Answer from the drawing. Dimensions are ordinates in mm from the lowest x, y and z of the part. Coordinates: 2 decimals unless noted, no trailing zeros. Order: outer loops, then holes, each group sorted by start corner. A loop starts at its lowest first (then second) coordinate and runs counter-clockwise, first axis right, second up. Notation, with made-up numbers: M 79.25,0 L 101.25,0 A20 cw 101.25,23 Z; hole C 69.25,79 d2. An arc over 180 degrees is marked long. Write each question's results on one line, items separated by ' | '.
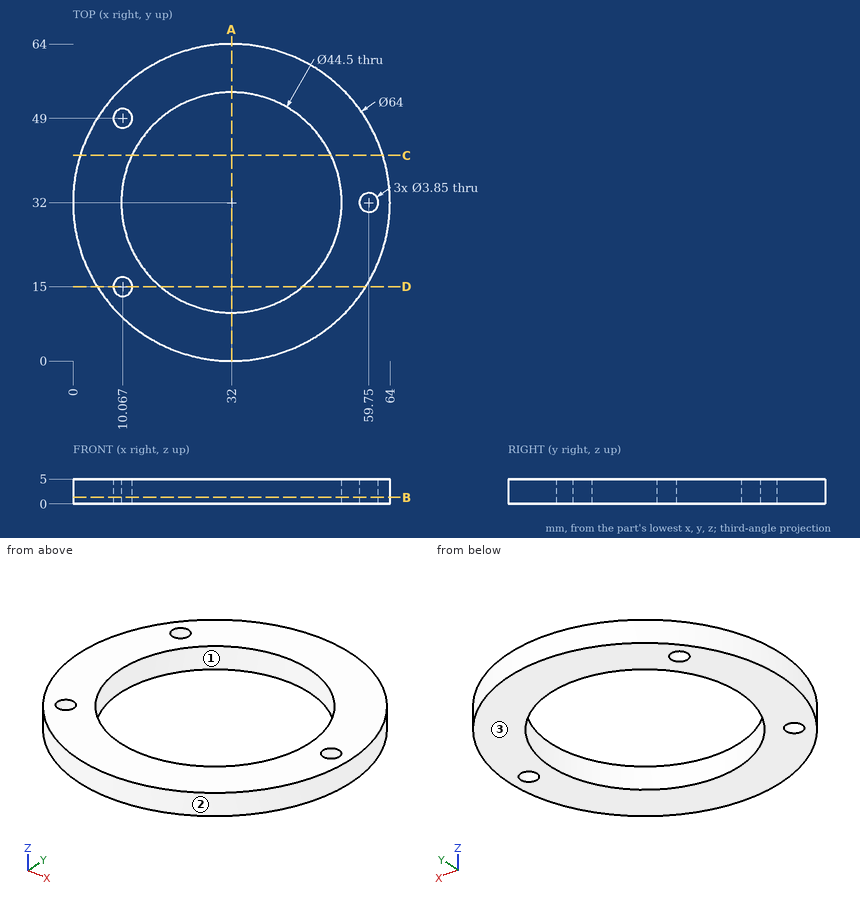
(1) Given pin 1 (2 mm diameter, centred on y = 23.5, z = 2.5, fed in from -X); pin 2 (3 mm diameter, centred on x = 39.5, z = 1, fed in from +Y); pin 3 (1 mm diameter, centred on y = 16, z = 3, fed in from +X), each flat-ended and moving along its own axis, determine where each tip first touches the part or whether it passes through.
Conclusion:
pin 1: x = 0.89 | pin 2: y = 63.43 | pin 3: x = 60
(2) The part is cut by section C-C, the plane y = 41.5. Write down the section's boundary in (x, z).
Conclusion:
outline: M 1.44,0 L 11.88,0 L 11.88,5 L 1.44,5 Z; M 52.12,0 L 62.56,0 L 62.56,5 L 52.12,5 Z
(3) The part is cut by section D-D, the plane y = 15. Write down the section's boundary in (x, z) (3 decimals).
Conclusion:
outline: M 4.889,0 L 8.142,0 L 8.142,5 L 4.889,5 Z; M 11.992,0 L 17.645,0 L 17.645,5 L 11.992,5 Z; M 46.355,0 L 59.111,0 L 59.111,5 L 46.355,5 Z
(4) Straight lines are drawn through the part: line 1 (X direction, y = 49.5, z = 3.5) (1 decimal); line 2 (Y direction, x = 45.5, z = 3.75); line 3 (Y direction, x = 43, z = 0.75). For each, find the intervals that lie inside material, in ascending order.
Conclusion:
line 1: 5.2 to 8.2, 11.9 to 18.3, 45.7 to 58.8 | line 2: 2.99 to 14.31, 49.69 to 61.01 | line 3: 1.95 to 12.66, 51.34 to 62.05
(5) The part is cut by section B-B, the plane z = 1.3. Write down the section's boundary in (x, y) (3 decimals), then the cut area to 3 significant figures.
Conclusion:
outline: C 32,32 d64; hole C 10.067,15 d3.85; hole C 10.067,49 d3.85; hole C 32,32 d44.5; hole C 59.75,32 d3.85 | area: 1,630 mm²
(6) The part is cut by section A-A, the plane x = 32. Write down the section's boundary in (y, z), then the cut area to 3 significant figures.
Conclusion:
outline: M 0,0 L 9.75,0 L 9.75,5 L 0,5 Z; M 54.25,0 L 64,0 L 64,5 L 54.25,5 Z | area: 97.5 mm²
(7) The mould has two halves that part along X. Classify the marked faces 1, 2 and 3: pulls with the +X half, pulls with the -X half, needs draft (parallel to the pull), parting line crosses it, or undercut.
Conclusion:
face 1: undercut | face 2: parting line crosses it | face 3: needs draft
